from build123d import *

# Parameters (mm, degrees)
F0_R     = 3.175
F1_DEPTH = 3.175
F2_R     = 1.5875
F3_DEPTH = 50.8
F4_R     = 3.175
F4_R_2   = 1.5875
F5_DEPTH = 3.175


with BuildPart() as f1:
    # F0 (on Right) → F1 (new body)
    with BuildSketch(Plane.YZ):
        Circle(F0_R)
    extrude(amount=F1_DEPTH)

    # F2 (on face) → F3 (join)
    with BuildSketch(Plane.YZ.offset(3.175)):
        Circle(F2_R)
    extrude(amount=F3_DEPTH)

    # F4 (on face) → F5 (join)
    with BuildSketch(Plane.YZ.offset(53.975)):
        Circle(F4_R)
        Circle(F4_R_2, mode=Mode.SUBTRACT)
        Circle(F4_R_2)
    extrude(amount=F5_DEPTH)


solid = f1.part
Could you check a few things on this model? Use its own coordinates, in mm. A direction names the side the tool comes from. Round coordinates to 2 decimals unless told otherwise and drop trailing zeros. Write each loop counter-clockwise with the first axis right and the second up, starting at its lowest first coordinate (ties: lowest second). Pieces come first, ordered by that corner, then holes. Notation, with made-up numbers: (71, 70) - (103, 70) arc R13 cw to (103, 92) - close; hole circle Ø3 at (34, 49.5). An arc over 180 degrees is marked (long way). Use a Markdown table: item, result.
Q1. I want a section at D-D (x = 47). List the corners of the cut face in (y, z) for me (1 decimal).
Output values:
| item | result |
|---|---|
| outline | circle Ø3.2 at (0, 0) |
Q2. For faces 1 (the flat face through (0, 0, 0)), 2 (the cylindrical face through (28.22, -0.34, -1.55)), which set-ups out of +Z, -Z, +X, -X, +Y, -Y let a thin tool reach every point of the face, with its end or its side?
Output values:
| item | result |
|---|---|
| face 1 | +Z, -Z, -X, +Y, -Y |
| face 2 | none |
Q3. Please list where these lines run through material, in increasing order: L1, parallel to X at y = -2, z = 1.25 (3 decimals); L2, parallel to Z at x = 18.5, y = 0; L3, parallel to Z at x = 31, y = -1.
Output values:
| item | result |
|---|---|
| L1 | 0 to 3.175, 53.975 to 57.15 |
| L2 | -1.59 to 1.59 |
| L3 | -1.23 to 1.23 |
Q4. I want a section at A-A (z = -2.25). List the corners of the cut face in (x, y) for me (3 decimals), plus the area to 3 significant figures.
Output values:
| item | result |
|---|---|
| outline | (0, -2.24) - (3.175, -2.24) - (3.175, 2.24) - (0, 2.24) - close; (53.975, -2.24) - (57.15, -2.24) - (57.15, 2.24) - (53.975, 2.24) - close |
| area | 28.4 mm2 |
Q5. For pin 1 (3 mm diameter, centred on x = 27, z = -1.5, fed in from +Y); pin 2 (3 mm diameter, centred on y = -2.5, z = -1.5, fed in from -X), each with a flat end and sliding along its axis, tell me the tip position at first contact or that it passes through.
Output values:
| item | result |
|---|---|
| pin 1 | y = 1.59 |
| pin 2 | x = 0 |
